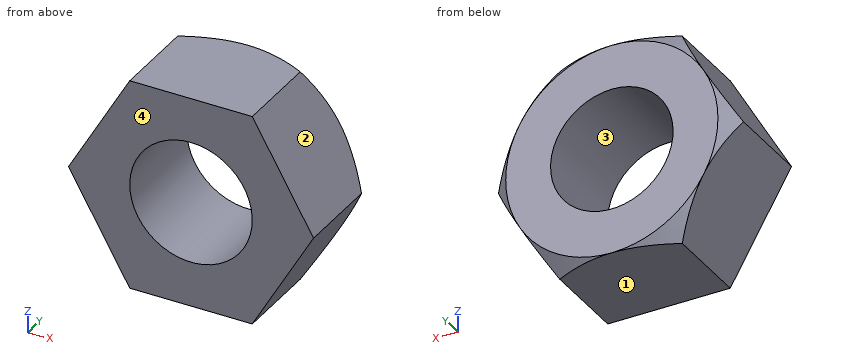
from build123d import *

# Parameters (mm, degrees)
BOSS_EXTRUDE1_DEPTH = 10
SKETCH2_OUTSIDE_W   = 56.658
SKETCH2_OUTSIDE_H   = 53.442
SKETCH2_OUTSIDE_R   = 10.392304845
CUT_EXTRUDE2_DEPTH  = 12
CUT_EXTRUDE2_DRAFT  = -45
CUT_EXTRUDE3_REACH  = 20.762
SKETCH3_R           = 6


with BuildPart() as part:
    # Sketch1 → Boss-Extrude1 (new body)
    with BuildSketch(Plane(origin=(0, 0, 0), x_dir=(1, 0, 0), z_dir=(0, 1, 0))):
        Polygon((6, -10.392304845), (12, 0), (6, 10.392304845), (-6, 10.392304845), (-12, 0), (-6, -10.392304845), align=None)
    extrude(amount=BOSS_EXTRUDE1_DEPTH)


with BuildPart() as cut_extrude2_tool:
    # Sketch2 outside → Cut-Extrude2 (with draft: the straight prism first)
    with BuildSketch(Plane(origin=(0, 10, 0), x_dir=(1, 0, 0), z_dir=(0, 1, 0))):
        Rectangle(SKETCH2_OUTSIDE_W, SKETCH2_OUTSIDE_H)
        Circle(SKETCH2_OUTSIDE_R, mode=Mode.SUBTRACT)
    extrude(amount=-CUT_EXTRUDE2_DEPTH)
    # Cut-Extrude2: the draft: its side faces are tilted about the plane it starts from
    cut_extrude2_sides = [cut_extrude2_tool.faces().sort_by_distance(p)[0] for p in [
        (0, 4, 26.721),
        (28.329, 4, 0),
        (0, 4, -26.721),
        (-28.329, 4, 0),
        (-10.392304845, 4, 0),
    ]]
    draft(cut_extrude2_sides, Plane(origin=(0, 10, 0), x_dir=(1, 0, 0), z_dir=(0, 1, 0)), CUT_EXTRUDE2_DRAFT)


with BuildPart() as part_1:
    add(part.part)

    # Cut-Extrude2: cut by cut_extrude2_tool
    add(cut_extrude2_tool.part, mode=Mode.SUBTRACT)

    # Sketch3 → Cut-Extrude3 (cut, up to next)
    with BuildSketch(Plane(origin=(0, 10, 0), x_dir=(1, 0, 0), z_dir=(0, 1, 0)), mode=Mode.PRIVATE) as cut_extrude3_sk1:
        with Locations(Location((0, 0, 0), (0, 0, 270))):
            Circle(SKETCH3_R)
    cut_extrude3_tool1 = extrude(cut_extrude3_sk1.sketch, amount=-CUT_EXTRUDE3_REACH, mode=Mode.PRIVATE) & part_1.part
    add(cut_extrude3_tool1.solids().sort_by_distance((0, 10, 0))[0], mode=Mode.SUBTRACT)


solid = part_1.part
Design review of the part built by this model. Coordinates are the model's own, in mm. Face numbers are marked on the shaded views. Coordinates: 2 decimals unless noted, no trailing zeros. Write each loop counter-clockwise with the first axis right and the second up, starting at its lowest first coordinate (ties: lowest second). Pieces come first, ordered by that corner, then holes. Notation, with made-up numbers: (73, 3.25) - (82, 3.25) arc R5 cw to (82, 9.25) - close; hole circle Ø8 at (79, 10.25). An arc over 180 degrees is marked (long way). Use one line per item in the form item = value.
Q1. Insertion check: pin 1 Ø4 at (y, z) = (4.5, 6.5) entering from +X; pin 2 Ø11 at (x, z) = (0, 0) entering from -Y. Each pin has a flat end and moves straight along its axis. Give the tip position at first contact, or say it passes through.
Taken from the geometry:
pin_1 = 9.4
pin_2 = through
Q2. The part is to be moulded in two halves that separate along Z. For the marked faces 1, 2, 3 and 4, say which applies: +Z half, -Z half, draft (parallel to the pull), parting line (faces both ways), or undercut.
Taken from the geometry:
face_1 = -Z half
face_2 = +Z half
face_3 = undercut
face_4 = draft
Q3. For probe 1 along Z at (x, y) = (9, 4.25); probe 2 along Z at (x, y) = (3.25, 8); probe 3 along Z at (x, y) = (-6.25, 2.25), list the stretches that pass through material, from the lowest coordinate up.
Taken from the geometry:
probe_1 = -5.2 to 5.2
probe_2 = -10.39 to -5.04, 5.04 to 10.39
probe_3 = -9.96 to 9.96
Q4. Consider section A-A (y = 5.5). Write out the cut boundary in (x, z), plus the area to 3 significant figures.
Taken from the geometry:
outline = (-12, 0) - (-6, -10.39) - (6, -10.39) - (12, 0) - (6, 10.39) - (-6, 10.39) - close; hole circle Ø12 at (0, 0)
area = 261 mm^2
